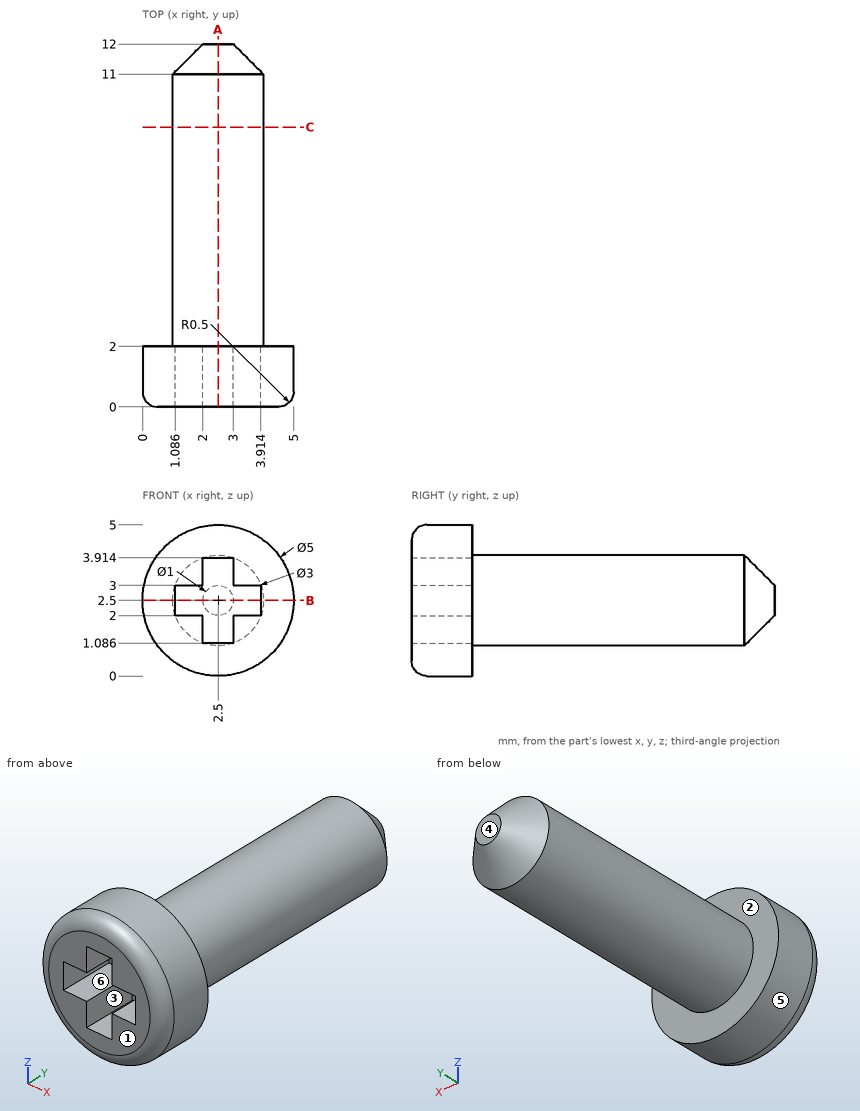
Answer from the drawing. Dimensions are ordinates in mm from the lowest x, y and z of the part. A direction names the side the tool comes from. Give positions to 0.01 mm unless a question says otherwise; leave off trailing zeros. Order: outer loops, then holes, each group sorted by start corner. A loop starts at its lowest first (then second) coordinate and runs counter-clockwise, first axis right, second up. Notation, with made-up numbers: (25.25, 36) - (79.25, 36) arc R15 cw to (79.25, 62) - close; hole circle Ø9 at (4.5, 66.25). An arc over 180 degrees is marked (long way). One line per item, written item: value. Start each with the question number.
1. Section A-A, the plane x = 2.5 is taken. Write down the section's boundary in (y, z).
2. Consider line 1 (X direction, y = 8.25, z = 2); line 2 (Y direction, x = 4.25, z = 2.1); line 3 (X direction, y = 1.5, z = 2.2). Determine where each line is inside the solid, lowest interval first.
3. Which of the six approach directions +Z, -Z, +X, -X, +Y, -Y give full straight-line access (tool end or side, diameter ignored) to the marked faces 1, 2 and 3?
4. Section B-B, the plane z = 2.5 is taken. Write down the section's boundary in (x, y).
5. Section C-C, the plane y = 9.25 is taken. Write down the section's boundary in (x, z).
6. Each of these flat-tipped pins is pushed along its axis until it touches: pin 1 Ø0.5 at (x, y) = (3.5, 0.5) entering from -Z (1 decimal); pin 2 Ø3 at (y, z) = (9.5, 4) entering from -X; pin 3 Ø1 at (y, z) = (0.5, 3.5) entering from -X. Where does it stop, or does it pass through?
7. For a pull along Z with two mould halves and no side action, classify the marked faces 4, 5 and 6 as released by +Z, released by -Z, zero draft, split by the parting line, or undercut.
Filled sheet:
1. outline: (0, 0.5) arc R0.5 ccw to (0.5, 0) - (2, 0) - (2, 1) - (11, 1) - (12, 2) - (12, 3) - (11, 4) - (2, 4) - (2, 5) - (0.5, 5) arc R0.5 ccw to (0, 4.5) - (0, 3.91) - (2, 3.91) - (2, 1.09) - (0, 1.09) - close
2. line 1: 1.09 to 3.91
2. line 2: 0 to 2
2. line 3: 0.02 to 1.09, 3.91 to 4.98
3. face 1: +Z, -Z, +X, -X, -Y
3. face 2: +Y
3. face 3: -Y
4. outline: (0, 0.5) arc R0.5 ccw to (0.5, 0) - (1.09, 0) - (1.09, 2) - (3.91, 2) - (3.91, 0) - (4.5, 0) arc R0.5 ccw to (5, 0.5) - (5, 2) - (4, 2) - (4, 11) - (3, 12) - (2, 12) - (1, 11) - (1, 2) - (0, 2) - close
5. outline: circle Ø3 at (2.5, 2.5)
6. pin 1: z = 0.1
6. pin 2: x = 1
6. pin 3: x = 0.05
7. face 4: zero draft
7. face 5: split by the parting line
7. face 6: undercut
